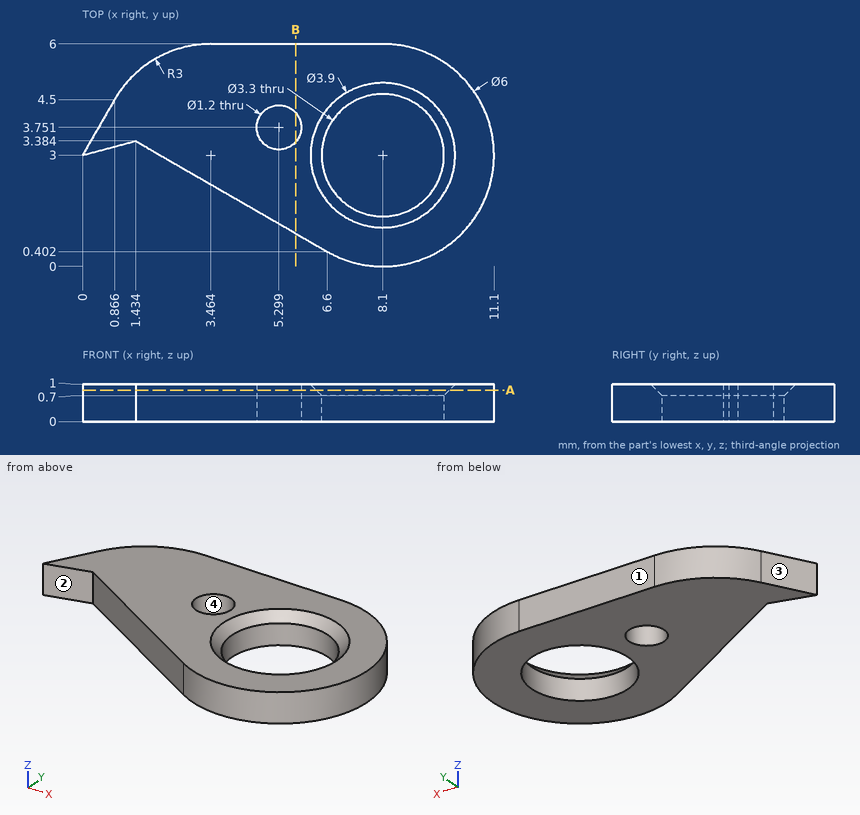
Design review of the part shown in the three views and the two pictorial views. Dimensions are in mm from the part's minimum x, y and z. Round coordinates to 2 decimals unless told otherwise and drop trailing zeros. Loops run counter-clockwise (first coordinate to the right, second up) from the corner with the lowest first, then second, coordinate; pieces in that order, holes last. Notation, with made-up numbers: M 20,81.5 L 69,81.5 A19 cw 69,91.5 Z; hole C 70.25,-26 d4. An arc over 180 degrees is marked long. Answer as a JSON object with one key per item and string values.
Item 1: The part is to be moulded in two halves that separate along X. For the marked faces 1, 2, 3 and 4, say which applies: pulls with the +X half, pulls with the -X half, needs draft (parallel to the pull), parting line crosses it, or undercut.
Answer sheet:
{"face 1": "needs draft", "face 2": "undercut", "face 3": "pulls with the -X half", "face 4": "undercut"}
Item 2: Wall thickness on L1, parallel to Y at x = 8.1, z = 0.5; L2, parallel to Y at x = 7.5, z = 0.15; L3, parallel to Y at x = 2.25, z = 0.75 (1 decimal): over which ranges is each line inside the solid? List them lowest first. Write a range as from..to.
Answer sheet:
{"L1": "y = 0..1.35, 4.65..6", "L2": "y = 0.06..1.46, 4.54..6", "L3": "y = 2.9..5.7"}
Item 3: We need section B-B on x = 5.75. Give the boundary of the cut face in (y, z) (1 decimal).
Answer sheet:
{"outline": "M 0.9,0 L 3.4,0 L 3.4,1 L 0.9,1 Z; M 4.1,0 L 6,0 L 6,1 L 4.1,1 Z"}
Item 4: We need section A-A on z = 0.85. State how many separate pieces and enclosed holes the cut face has, and give its area (3 significant figures).
Answer sheet:
{"separate pieces": "1", "enclosed holes": "2", "area": "33.8 mm^2"}
